Here's how the part is built. I have some questions about the finished solid (model axes, mm). Face numbers are marked on the shaded views. A direction names the side the tool comes from. Round coordinates to 2 decimals unless told otherwise and drop trailing zeros. Write each loop counter-clockwise with the first axis right and the second up, starting at its lowest first coordinate (ties: lowest second). Pieces come first, ordered by that corner, then holes. Notation, with made-up numbers: (13, 58) - (21, 58) arc R22 ccw to (21, 74) - close; hole circle Ø3 at (81, -8.75). An arc over 180 degrees is marked (long way). Use one line per item in the form item = value. Start each with the question number.
1. I want a section at B-B, the plane z = 0. List the corners of the cut face in (x, y) for me.
2. Which directions (+Z, -Z, +X, -X, +Y, -Y) give clear straight access to the entire face, cutting with the end or side of a thin tool? Please do the marked faces 5, 6 and 7.
3. We'd pull the mould along Z, two halves only. Please class the marked faces 1, 2, 3 and 4: +Z half, -Z half, draft (parallel to the pull), parting line (faces both ways), or undercut.
4. If I drill on line 1 along Y through (x, z) = (-20, -5); line 2 along Y through (x, z) = (7.5, -2); line 3 along Z through (x, y) = (-24, -6.5), over which ranges is the centre line in solid material (lowest first)?
5. Will these pins go through, and if not, where does the flat tip stop? pin 1 (1 mm diameter, centred on y = -19.5, z = 15.5, fed in from +X); pin 2 (2 mm diameter, centred on x = 11.5, z = 3, fed in from +Y); pin 3 (4 mm diameter, centred on x = -3, y = 10, fed in from +Z).
6. I want a section at C-C, the plane x = 13. List the corners of the cut face in (y, z) for me, plus the area to 3 significant figures.
7. I want a section at D-D, the plane x = 0. List the corners of the cut face in (y, z) for me.
8. I want a section at A-A, the plane y = -21. List the corners of the cut face in (x, z) for me, plus the area to 3 significant figures.
```python
from build123d import *

# Parameters (mm, degrees)
F0_W     = 69.888253
F0_H     = 54.705635
F1_DEPTH = 41.656
F2_T     = -2.54
F3_R     = 9.833618
F4_DEPTH = 75.184


with BuildPart() as f1:
    # F0 (on Front) → F1 (new body)
    with BuildSketch(Plane.XZ):
        with Locations((0.963976, -1.56646)):
            Rectangle(F0_W, F0_H)
    extrude(amount=F1_DEPTH)

    # F2
    f2_openings = [f1.faces().sort_by_distance(p)[0] for p in [
        (35.908103, -20.828, -1.56646),
    ]]
    offset(amount=F2_T, openings=f2_openings)

    # F3 (on face) → F4 (join)
    with BuildSketch(Plane(origin=(0, 0, 0), x_dir=(-1, 0, 0), z_dir=(0, 1, 0))):
        Circle(F3_R)
    extrude(amount=F4_DEPTH)


solid = f1.part
```
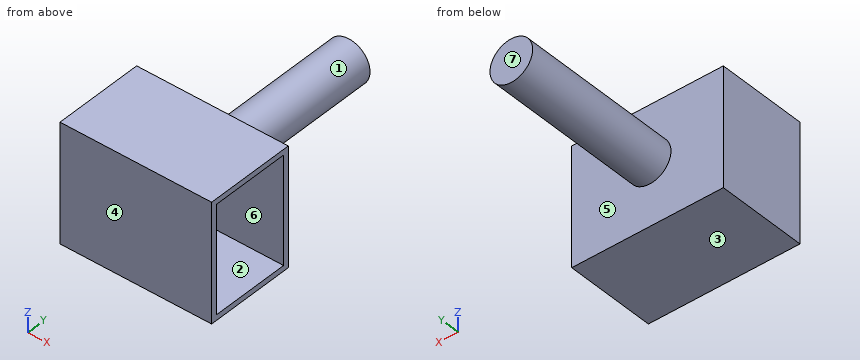
Model answer:
q1.outline = (-33.98, -41.66) - (35.91, -41.66) - (35.91, -39.12) - (-31.44, -39.12) - (-31.44, -2.54) - (35.91, -2.54) - (35.91, 0) - (9.83, 0) - (9.83, 75.18) - (-9.83, 75.18) - (-9.83, 0) - (-33.98, 0) - close
q2.face_5 = +Y
q2.face_6 = +X
q2.face_7 = +Z, -Z, +X, -X, +Y
q3.face_1 = parting line
q3.face_2 = undercut
q3.face_3 = -Z half
q3.face_4 = draft
q4.line_1 = -41.66 to -39.12, -2.54 to 0
q4.line_2 = -41.66 to -39.12, -2.54 to 75.18
q4.line_3 = -28.92 to -26.38, 23.25 to 25.79
q5.pin_1 = -31.44
q5.pin_2 = 0
q5.pin_3 = 9.78
q6.outline = (-41.66, -28.92) - (0, -28.92) - (0, 25.79) - (-41.66, 25.79) - close; hole (-39.12, -26.38) - (-2.54, -26.38) - (-2.54, 23.25) - (-39.12, 23.25) - close
q6.area = 464 mm2
q7.outline = (-41.66, -28.92) - (0, -28.92) - (0, -9.83) - (75.18, -9.83) - (75.18, 9.83) - (0, 9.83) - (0, 25.79) - (-41.66, 25.79) - close; hole (-39.12, -26.38) - (-2.54, -26.38) - (-2.54, 23.25) - (-39.12, 23.25) - close
q8.outline = (-33.98, -28.92) - (35.91, -28.92) - (35.91, -26.38) - (-31.44, -26.38) - (-31.44, 23.25) - (35.91, 23.25) - (35.91, 25.79) - (-33.98, 25.79) - close
q8.area = 481 mm2
